from build123d import *

# Parameters (mm, degrees)
SKETCH1_W           = 90
SKETCH1_H           = 100
SKETCH1_W_2         = 85
SKETCH1_H_2         = 95
BOSS_EXTRUDE1_DEPTH = 30
SKETCH2_W           = 2.5
SKETCH2_H           = 10
BOSS_EXTRUDE2_DEPTH = 10
REVOLVE1_ANGLE      = 180
CUT_EXTRUDE1_DEPTH  = 76


with BuildPart() as part:
    # Sketch1 → Boss-Extrude1 (new body)
    with BuildSketch(Plane(origin=(0, 0, 0), x_dir=(1, 0, 0), z_dir=(0, 1, 0))):
        Rectangle(SKETCH1_W, SKETCH1_H)
        Rectangle(SKETCH1_W_2, SKETCH1_H_2, mode=Mode.SUBTRACT)
    extrude(amount=BOSS_EXTRUDE1_DEPTH)

    # Sketch2 → Boss-Extrude2 (add)
    with BuildSketch(Plane.XZ):
        Polygon((-42.5, 47.5), (-42.5, 50), (-45, 50), (-45, 40), (-42.5, 40), align=None)
        Polygon((42.5, 47.5), (42.5, 50), (45, 50), (45, 40), (42.5, 40), align=None)
        Polygon((-42.5, -47.5), (-42.5, -40), (-45, -40), (-45, -50), (-42.5, -50), align=None)
        with Locations((43.75, -45)):
            Rectangle(SKETCH2_W, SKETCH2_H)
    extrude(amount=BOSS_EXTRUDE2_DEPTH)

    # Sketch4 → Revolve1 (revolve)
    with BuildSketch(Plane(origin=(0, 30, 0), x_dir=(1, 0, 0), z_dir=(0, 1, 0))):
        Polygon((45, 50), (45, -50), (0, -50), (0, -47.5), (42.5, -47.5), (42.5, 47.5), (0, 47.5), (0, 50), align=None)
    revolve(axis=Axis((0, 30, -57.663927553), (0, 0, 1)), revolution_arc=REVOLVE1_ANGLE)

    # Sketch5 → Cut-Extrude1 (cut, through all)
    with BuildSketch(Plane(origin=(0, 0, 0), x_dir=(1, 0, 0), z_dir=(0, 1, 0))):
        Polygon((30, 30), (-90, 30), (-90, -30), (30, -30), (30, -20), (-80, -20), (-80, -10), (-80, 10), (-80, 20), (30, 20), align=None)
    extrude(amount=CUT_EXTRUDE1_DEPTH, mode=Mode.SUBTRACT)


solid = part.part
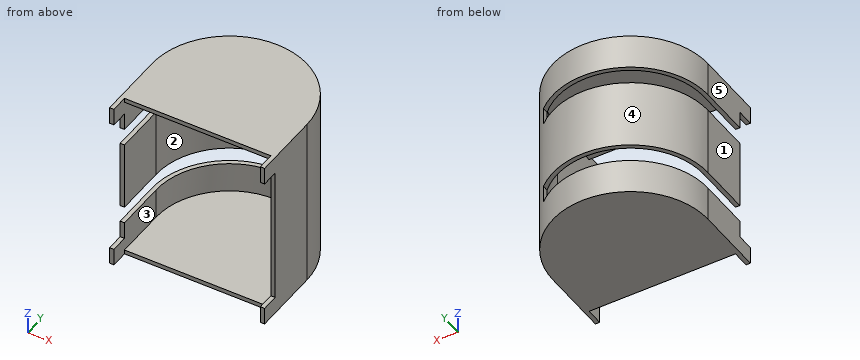
For this review, take the finished solid that the model builds, in its own axes (mm). Face numbers are marked on the shaded views. A direction names the side the tool comes from. Coordinates: 2 decimals unless noted, no trailing zeros. Order: outer loops, then holes, each group sorted by start corner. A loop starts at its lowest first (then second) coordinate and runs counter-clockwise, first axis right, second up. Notation, with made-up numbers: (76.25, -11.5) - (96.25, -11.5) arc R3 cw to (96.25, -6.5) - close; hole circle Ø1 at (11.25, 17). An arc over 180 degrees is marked (long way). Answer as CSV lines item,"result". Start each with the question number.
1) Add section D-D (y = 57). State the section outline as (x, z) points.
2) To check wall thickness, follow line 1 along Z through (x, y) = (-29.5, 61); line 2 along X through (y, z) = (22, 42); line 3 along Z through (x, y) = (15, 54.5). State the ranges of each line that lie inside material, in increasing order. Write a range as [from, to].
3) Insertion check: P1, Ø3, axis at x = -0.5, z = -48.5, coming from the -Y side; P2, Ø1.5, axis at x = 24.5, z = -6, coming from the +Y side; P3, Ø1, axis at y = 38, z = -19, coming from the +X side. Each pin has a flat end and moves straight along its axis. Give the tip position at first contact, or say it passes through.
4) Add section B-B (x = 0). State the section outline as (y, z) points, then the cut area to 4 significant figures.
5) Machinability: for the marked faces 1 and 2, which of the approach directions +Z, -Z, +X, -X, +Y, -Y give a long, thin tool a straight path to every point of the face, cutting with its end or side? Answer none if there is none.
6) Draft analysis for pull direction X (two halves, no side actions). For the marked faces 3, 4 and 5, state which applies: +X half, -X half, draft (parallel to the pull), parting line (faces both ways), or undercut.
7) Add section A-A (y = 21.5). State the section outline as (x, z) points, then the cut area to 3 significant figures.
8) Add section C-C (z = -23.5). State the section outline as (x, y) points, then the cut area to 3 significant figures.
Result:
1,outline,"(-36, -50) - (36, -50) - (36, 50) - (-36, 50) - (-36, 30) - (-32.82, 30) - (-32.82, 47.5) - (32.82, 47.5) - (32.82, -47.5) - (-32.82, -47.5) - (-32.82, -30) - (-36, -30) - close; (-36, -20) - (-32.82, -20) - (-32.82, 20) - (-36, 20) - close"
2,line 1,"[-50, -30], [-20, 20], [30, 50]"
2,line 2,"[-45, -42.5], [42.5, 45]"
2,line 3,"[-50, -47.5], [47.5, 50]"
3,P1,"y = 0"
3,P2,"y = 68.22"
3,P3,"x = 44.37"
4,outline,"(0, -50) - (75, -50) - (75, -30) - (72.5, -30) - (72.5, -47.5) - (0, -47.5) - close; (0, 47.5) - (72.5, 47.5) - (72.5, 30) - (75, 30) - (75, 50) - (0, 50) - close; (72.5, -20) - (75, -20) - (75, 20) - (72.5, 20) - close"
4,area,"562.5 mm^2"
5,face 1,"+Z, -Z, -X, +Y, -Y"
5,face 2,"-Y"
6,face 3,"undercut"
6,face 4,"parting line"
6,face 5,"-X half"
7,outline,"(-45, -50) - (45, -50) - (45, 50) - (-45, 50) - (-45, 30) - (-42.5, 30) - (-42.5, 47.5) - (42.5, 47.5) - (42.5, -47.5) - (-42.5, -47.5) - (-42.5, -30) - (-45, -30) - close; (-45, -20) - (-42.5, -20) - (-42.5, 20) - (-45, 20) - close"
7,area,"875 mm^2"
8,outline,"(30, 60.1) arc R42.5 cw to (42.5, 30) - (42.5, 0) - (45, 0) - (45, 30) arc R45 ccw to (30, 63.54) - close"
8,area,"164 mm^2"
